Here's how the part is built. I have some questions about the finished solid (model axes, mm). Face numbers are marked on the shaded views. A direction names the side the tool comes from. Coordinates: 2 decimals unless noted, no trailing zeros. Write each loop counter-clockwise with the first axis right and the second up, starting at its lowest first coordinate (ties: lowest second). Pieces come first, ordered by that corner, then holes. Notation, with made-up numbers: (81.5, 27.5) - (102.5, 27.5) arc R12 cw to (102.5, 43.5) - close; hole circle Ø10 at (67, 0). An arc over 180 degrees is marked (long way). Answer in a Markdown table with one row per item. Add a question column.
Item 1: I'm going to push flat-ended pins straight in: pin 1 (1.7 mm diameter, centred on x = -20, z = 13, fed in from -Y); pin 2 (1.5 mm diameter, centred on y = 19.5, z = 9.5, fed in from +X); pin 3 (1.5 mm diameter, centred on x = 18.5, z = 12, fed in from -Y). Where does each tip first touch, or does it pass through?
Item 2: Which directions (+Z, -Z, +X, -X, +Y, -Y) give clear straight access to the entire face, cutting with the end or side of a thin tool? Please do the marked faces 5, 6 and 7.
Item 3: Imagine slicing it at D-D (x = 39.5). Please give me the cut outline in (y, z).
Item 4: Imagine slicing it at A-A (y = 0). Please give me the cut outline in (x, z), plus the area to 3 significant figures.
Item 5: If I drill on probe 1 along Y at (x, z) = (0, 8); probe 2 along Y at (x, z) = (-1, 7.25); probe 3 along X at (y, z) = (31.5, 2.25), over which ranges is the centre line in solid material (lowest first)? Write a range as from..to.
Item 6: Imagine slicing it at B-B (x = 0). Please give me the cut outline in (y, z).
Item 7: Imagine slicing it at C-C (z = 18.25). State how many separate pieces and enclosed holes the cut face has, plus the area to 3 significant figures.
Item 8: We'd pull the mould along Y, two halves only. Please class the marked faces 1, 2, 3 and 4: +Y half, -Y half, draft (parallel to the pull), parting line (faces both ways), or undercut.
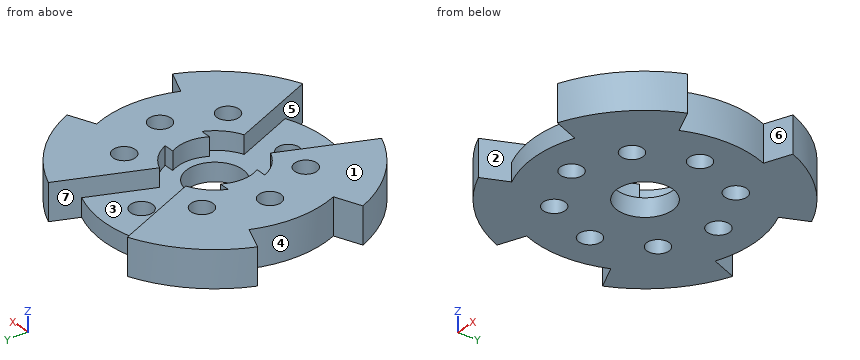
from build123d import *

# Parameters (mm, degrees)
SKETCH1_R             = 6
BOSS_EXTRUDE1_DEPTH   = 20
BOSS_EXTRUDE1_2_DEPTH = 20
SKETCH1_3_R           = 6
SKETCH1_3_R_2         = 15
BOSS_EXTRUDE2_DEPTH   = 10


with BuildPart() as part:
    # Sketch1 → Boss-Extrude1 (new body)
    with BuildSketch(Plane.XY):
        with BuildLine():
            Line((17.320508076, -10), (22.912878475, -10))
            ThreePointArc((22.912878475, -10), (17.510562404, -17.843211715), (9.567085809, -23.096988313))
            Line((9.567085809, -23.096988313), (28.701257427, -69.290964938))
            ThreePointArc((28.701257427, -69.290964938), (53.033008589, -53.033008589), (69.290964938, -28.701257427))
            Line((69.290964938, -28.701257427), (55.432771951, -22.961005942))
            ThreePointArc((55.432771951, -22.961005942), (60, 0), (55.432771951, 22.961005942))
            Line((55.432771951, 22.961005942), (69.290964938, 28.701257427))
            ThreePointArc((69.290964938, 28.701257427), (53.033008589, 53.033008589), (28.701257427, 69.290964938))
            Line((28.701257427, 69.290964938), (9.567085809, 23.096988313))
            ThreePointArc((9.567085809, 23.096988313), (17.510562404, 17.843211715), (22.912878475, 10))
            Line((22.912878475, 10), (17.320508076, 10))
            ThreePointArc((17.320508076, 10), (20, 0), (17.320508076, -10))
        make_face()
        with Locations((28.284271247, -28.284271247)):
            Circle(SKETCH1_R, mode=Mode.SUBTRACT)
        with Locations((40, 0)):
            Circle(SKETCH1_R, mode=Mode.SUBTRACT)
        with Locations((28.284271247, 28.284271247)):
            Circle(SKETCH1_R, mode=Mode.SUBTRACT)
    extrude(amount=BOSS_EXTRUDE1_DEPTH)



with BuildPart() as body_2:
    # Sketch1 → Boss-Extrude1 2 (new body)
    with BuildSketch(Plane.XY):
        with BuildLine():
            ThreePointArc((-28.701257427, -69.290964938), (-53.033008589, -53.033008589), (-69.290964938, -28.701257427))
            Line((-69.290964938, -28.701257427), (-55.432771951, -22.961005942))
            ThreePointArc((-55.432771951, -22.961005942), (-60, 0), (-55.432771951, 22.961005942))
            Line((-55.432771951, 22.961005942), (-69.290964938, 28.701257427))
            ThreePointArc((-69.290964938, 28.701257427), (-53.033008589, 53.033008589), (-28.701257427, 69.290964938))
            Line((-28.701257427, 69.290964938), (-9.567085809, 23.096988313))
            ThreePointArc((-9.567085809, 23.096988313), (-17.510562404, 17.843211715), (-22.912878475, 10))
            Line((-22.912878475, 10), (-17.320508076, 10))
            ThreePointArc((-17.320508076, 10), (-20, 0), (-17.320508076, -10))
            Line((-17.320508076, -10), (-22.912878475, -10))
            ThreePointArc((-22.912878475, -10), (-17.510562404, -17.843211715), (-9.567085809, -23.096988313))
            Line((-9.567085809, -23.096988313), (-28.701257427, -69.290964938))
        make_face()
        with Locations((-28.284271247, 28.284271247)):
            Circle(SKETCH1_R, mode=Mode.SUBTRACT)
        with Locations((-40, 0)):
            Circle(SKETCH1_R, mode=Mode.SUBTRACT)
        with Locations((-28.284271247, -28.284271247)):
            Circle(SKETCH1_R, mode=Mode.SUBTRACT)
    extrude(amount=BOSS_EXTRUDE1_2_DEPTH)


with BuildPart() as part_1:
    add(part.part)

    add(body_2.part)  # Boss-Extrude2 merges body 2
    # Sketch1_3 → Boss-Extrude2 (add)
    with BuildSketch(Plane.XY):
        with BuildLine():
            ThreePointArc((17.320508076, -10), (20, 0), (17.320508076, 10))
            Line((17.320508076, 10), (22.912878475, 10))
            ThreePointArc((22.912878475, 10), (17.510562404, 17.843211715), (9.567085809, 23.096988313))
            Line((9.567085809, 23.096988313), (22.961005942, 55.432771951))
            ThreePointArc((22.961005942, 55.432771951), (0, 60), (-22.961005942, 55.432771951))
            Line((-22.961005942, 55.432771951), (-9.567085809, 23.096988313))
            ThreePointArc((-9.567085809, 23.096988313), (-17.510562404, 17.843211715), (-22.912878475, 10))
            Line((-22.912878475, 10), (-17.320508076, 10))
            ThreePointArc((-17.320508076, 10), (-20, 0), (-17.320508076, -10))
            Line((-17.320508076, -10), (-22.912878475, -10))
            ThreePointArc((-22.912878475, -10), (-17.510562404, -17.843211715), (-9.567085809, -23.096988313))
            Line((-9.567085809, -23.096988313), (-22.961005942, -55.432771951))
            ThreePointArc((-22.961005942, -55.432771951), (0, -60), (22.961005942, -55.432771951))
            Line((22.961005942, -55.432771951), (9.567085809, -23.096988313))
            ThreePointArc((9.567085809, -23.096988313), (17.510562404, -17.843211715), (22.912878475, -10))
            Line((22.912878475, -10), (17.320508076, -10))
        make_face()
        with Locations((0, -40)):
            Circle(SKETCH1_3_R, mode=Mode.SUBTRACT)
        Circle(SKETCH1_3_R_2, mode=Mode.SUBTRACT)
        with Locations((0, 40)):
            Circle(SKETCH1_3_R, mode=Mode.SUBTRACT)
    extrude(amount=BOSS_EXTRUDE2_DEPTH)


solid = part_1.part
Here are the results:
| question | item | result |
|---|---|---|
| 1 | pin 1 | stops at y = -50.34 |
| 1 | pin 2 | stops at x = 57 |
| 1 | pin 3 | stops at y = -46.47 |
| 2 | face 5 | +Z, -Y |
| 2 | face 6 | +Z, -Z, +X |
| 2 | face 7 | +Z, +Y |
| 3 | outline | (-63.76, 0) - (-5.98, 0) - (-5.98, 20) - (-63.76, 20) - close; (5.98, 0) - (63.76, 0) - (63.76, 20) - (5.98, 20) - close |
| 4 | outline | (-60, 0) - (-46, 0) - (-46, 20) - (-60, 20) - close; (-34, 0) - (-15, 0) - (-15, 10) - (-20, 10) - (-20, 20) - (-34, 20) - close; (15, 0) - (34, 0) - (34, 20) - (20, 20) - (20, 10) - (15, 10) - close; (46, 0) - (60, 0) - (60, 20) - (46, 20) - close |
| 4 | area | 1,220 mm2 |
| 5 | probe 1 | y = -60..-46, -34..-15, 15..34, 46..60 |
| 5 | probe 2 | y = -59.99..-45.92, -34.08..-14.97, 14.97..34.08, 45.92..59.99 |
| 5 | probe 3 | x = -68.06..-33.35, -23.22..23.22, 33.35..68.06 |
| 6 | outline | (-60, 0) - (-46, 0) - (-46, 10) - (-60, 10) - close; (-34, 0) - (-15, 0) - (-15, 10) - (-34, 10) - close; (15, 0) - (34, 0) - (34, 10) - (15, 10) - close; (46, 0) - (60, 0) - (60, 10) - (46, 10) - close |
| 7 | separate pieces | 2 |
| 7 | enclosed holes | 6 |
| 7 | area | 9,720 mm2 |
| 8 | face 1 | draft |
| 8 | face 2 | -Y half |
| 8 | face 3 | undercut |
| 8 | face 4 | undercut |
